```python
from build123d import *

# Parameters (mm, degrees)
F0_R     = 2.5
F0_R_2   = 3
F0_W     = 13
F0_H     = 19
F0_R_3   = 10
F0_R_4   = 5
F1_DEPTH = 8
F2_R     = 30
F3_R     = 2


with BuildPart() as f1:
    # F0 (on Top) → F1 (new body)
    with BuildSketch(Plane.XY):
        with BuildLine():
            Line((-105, -88.5), (-105, -140))
            Line((-105, -140), (105, -140))
            Line((105, -140), (105, -88.5))
            Line((105, -88.5), (75, -88.5))
            Line((75, -88.5), (75, -16.5))
            Line((75, -16.5), (105, -16.5))
            Line((105, -16.5), (105, 0))
            ThreePointArc((105, 0), (85.327217, 78.134499), (31, 137.637204))
            ThreePointArc((31, 137.637204), (0, 146.835757), (-31, 137.637204))
            ThreePointArc((-31, 137.637204), (-85.327217, 78.134499), (-105, 0))
            Line((-105, 0), (-105, -16.5))
            Line((-105, -16.5), (-75, -16.5))
            Line((-75, -16.5), (-75, -88.5))
            Line((-75, -88.5), (-105, -88.5))
        make_face()
        with Locations((-65.5, -60.5)):
            Circle(F0_R, mode=Mode.SUBTRACT)
        with Locations((-59.1, -60.5)):
            Circle(F0_R, mode=Mode.SUBTRACT)
        with Locations((-52.7, -60.5)):
            Circle(F0_R, mode=Mode.SUBTRACT)
        with Locations((-65.5, -44.5)):
            Circle(F0_R, mode=Mode.SUBTRACT)
        with Locations((-59.1, -44.5)):
            Circle(F0_R, mode=Mode.SUBTRACT)
        with Locations((-52.7, -44.5)):
            Circle(F0_R, mode=Mode.SUBTRACT)
        with Locations((-46.3, -60.5)):
            Circle(F0_R, mode=Mode.SUBTRACT)
        with Locations((-39.9, -60.5)):
            Circle(F0_R, mode=Mode.SUBTRACT)
        with Locations((-46.3, -44.5)):
            Circle(F0_R, mode=Mode.SUBTRACT)
        with Locations((-39.9, -44.5)):
            Circle(F0_R, mode=Mode.SUBTRACT)
        with Locations((-10, -45)):
            Circle(F0_R_2, mode=Mode.SUBTRACT)
        with Locations((-46.5, -0.5)):
            Rectangle(F0_W, F0_H, mode=Mode.SUBTRACT)
        with Locations((0, -63)):
            Circle(F0_R_3, mode=Mode.SUBTRACT)
        with Locations((10, -45)):
            Circle(F0_R_2, mode=Mode.SUBTRACT)
        with Locations((39.9, -60.5)):
            Circle(F0_R, mode=Mode.SUBTRACT)
        with Locations((46.3, -60.5)):
            Circle(F0_R, mode=Mode.SUBTRACT)
        with Locations((39.9, -44.5)):
            Circle(F0_R, mode=Mode.SUBTRACT)
        with Locations((46.3, -44.5)):
            Circle(F0_R, mode=Mode.SUBTRACT)
        with Locations((52.7, -60.5)):
            Circle(F0_R, mode=Mode.SUBTRACT)
        with Locations((59.1, -60.5)):
            Circle(F0_R, mode=Mode.SUBTRACT)
        with Locations((65.5, -60.5)):
            Circle(F0_R, mode=Mode.SUBTRACT)
        with Locations((52.7, -44.5)):
            Circle(F0_R, mode=Mode.SUBTRACT)
        with Locations((59.1, -44.5)):
            Circle(F0_R, mode=Mode.SUBTRACT)
        with Locations((65.5, -44.5)):
            Circle(F0_R, mode=Mode.SUBTRACT)
        with Locations((-7.75, 70)):
            Circle(F0_R_2, mode=Mode.SUBTRACT)
        with Locations((-50, 85)):
            Circle(F0_R, mode=Mode.SUBTRACT)
        with Locations((-30, 104.595918)):
            Circle(F0_R, mode=Mode.SUBTRACT)
        with Locations((-7.75, 90)):
            Circle(F0_R, mode=Mode.SUBTRACT)
        with Locations((-14, 118)):
            Circle(F0_R, mode=Mode.SUBTRACT)
        with Locations((0, 50)):
            Circle(F0_R_4, mode=Mode.SUBTRACT)
        with Locations((7.75, 70)):
            Circle(F0_R_2, mode=Mode.SUBTRACT)
        with Locations((7.75, 90)):
            Circle(F0_R, mode=Mode.SUBTRACT)
        with Locations((50, 85)):
            Circle(F0_R, mode=Mode.SUBTRACT)
        with Locations((30, 104.595918)):
            Circle(F0_R, mode=Mode.SUBTRACT)
        with Locations((14, 118)):
            Circle(F0_R, mode=Mode.SUBTRACT)
    extrude(amount=F1_DEPTH)

    # F2
    f2_edges = [f1.edges().sort_by_distance(p)[0] for p in [
        (-105, -140, 4),
        (105, -140, 4),
    ]]
    fillet(f2_edges, radius=F2_R)

    # F3
    f3_edges = [f1.edges().sort_by_distance(p)[0] for p in [
        (-75, -16.5, 4),
        (-105, -16.5, 4),
        (-75, -88.5, 4),
        (-105, -88.5, 4),
        (75, -16.5, 4),
        (105, -16.5, 4),
        (75, -88.5, 4),
        (105, -88.5, 4),
    ]]
    fillet(f3_edges, radius=F3_R)


solid = f1.part
```
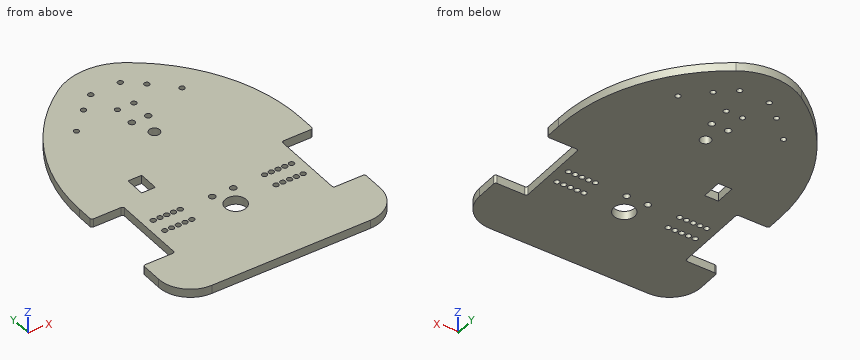
Work out the finished part from the listing and answer in its coordinate system (mm). Coordinates: 2 decimals unless noted, no trailing zeros. Write each loop counter-clockwise with the first axis right and the second up, starting at its lowest first coordinate (ties: lowest second). Pieces come first, ordered by that corner, then holes. Notation, with made-up numbers: (-8, -3.5) - (41, -3.5) arc R17 ccw to (41, 21.5) - close; hole circle Ø10 at (-28, 1). An arc over 180 degrees is marked (long way). Answer as a JSON object with one key per item and string values.
Q1. Consider L1, parallel to Y at x = 65.5, z = 2.5; L2, parallel to Y at x = 64, z = 4.75; L3, parallel to Y at x = -7.75, z = 5.25. Determine where each line is inside the solid, lowest interval first. Write a range as from..to.
Results list:
{"L1": "y = -140..-63, -58..-47, -42..107.12", "L2": "y = -140..-62.5, -58.5..-46.5, -42.5..108.85", "L3": "y = -140..-69.32, -56.68..-46.98, -43.02..67, 73..87.5, 92.5..146.3"}
Q2. Given pin 1 Ø2 at (y, z) = (-68, 2.5) entering from -X; pin 2 Ø1 at (y, z) = (108, 7) entering from +X; pin 3 Ø1 at (y, z) = (47.5, 3) entering from -X, each flat-ended and moving along its own axis, determine where each tip first touches the part or whether it passes through.
Results list:
{"pin 1": "stops at x = -75", "pin 2": "stops at x = 65.17", "pin 3": "stops at x = -98.16"}
Q3. Find section B-B (y = 28.5). Write down the section's boundary in (x, z).
Results list:
{"outline": "(-102.52, 0) - (102.52, 0) - (102.52, 8) - (-102.52, 8) - close"}
Q4. Find section A-A (y = 70). Write down the section's boundary in (x, z), plus the area to 3 significant figures.
Results list:
{"outline": "(-89.42, 0) - (-10.75, 0) - (-10.75, 8) - (-89.42, 8) - close; (-4.75, 0) - (4.75, 0) - (4.75, 8) - (-4.75, 8) - close; (10.75, 0) - (89.42, 0) - (89.42, 8) - (10.75, 8) - close", "area": "1,330 mm^2"}
Q5. Find section C-C (z = 2.75). State how many separate pieces and enclosed holes the cut face has, plus the area to 3 significant figures.
Results list:
{"separate pieces": "1", "enclosed holes": "35", "area": "46,600 mm^2"}
